Input: part model. Units: mm. Frame: model coordinates. A direction names the side the tool comes from. Coordinates: 2 decimals unless noted, no trailing zeros. Write each loop counter-clockwise with the first axis right and the second up, starting at its lowest first coordinate (ties: lowest second). Pieces come first, ordered by that corner, then holes. Notation, with made-up numbers: M -22,66.25 L -14,66.25 A12 cw -14,74.25 Z; hole C 79,27.25 d8. An arc over 180 degrees is marked long. Answer as a JSON object with one key per item and string values. Group by question number.
from build123d import *

# Parameters (mm, degrees)
F0_W      = 125
F0_H      = 200
F1_DEPTH  = 50
F2_W      = 50
F2_H      = 70
F3_DEPTH  = 35
F5_DEPTH  = 50
F6_R      = 20
F7_DEPTH  = 50.001
F9_DEPTH  = 30
F10_W     = 75
F10_H     = 25
F11_DEPTH = 200.001
F12_W     = 40
F12_H     = 50
F13_DEPTH = 20
F15_DEPTH = 40


with BuildPart() as f1:
    # F0 (on Top) → F1 (new body)
    with BuildSketch(Plane.XY):
        with Locations((-0.529949, 21.220052)):
            Rectangle(F0_W, F0_H)
    extrude(amount=F1_DEPTH)

    # F2 (on face) → F3 (join)
    with BuildSketch(Plane.XY.offset(50)):
        with Locations((-38.029949, 86.220052)):
            Rectangle(F2_W, F2_H)
    extrude(amount=F3_DEPTH)

    # F4 (on face) → F5 (join)
    with BuildSketch(Plane.YZ.offset(-13.029949)):
        with BuildLine():
            Line((51.220052, 85), (121.220052, 85))
            ThreePointArc((121.220052, 85), (86.220052, 120), (51.220052, 85))
        make_face()
    extrude(amount=-F5_DEPTH)

    # F6 (on face) → F7 (cut, through all)
    with BuildSketch(Plane.YZ.offset(-13.029949)):
        with Locations((86.220052, 85)):
            Circle(F6_R)
    extrude(amount=-F7_DEPTH, mode=Mode.SUBTRACT)

    # F8 (on face) → F9 (join)
    with BuildSketch(Plane(origin=(-63.029949, 0, 0), x_dir=(0, -1, 0), z_dir=(-1, 0, 0))):
        with BuildLine():
            Line((-51.220052, 50), (8.779948, 50))
            Line((8.779948, 50), (-63.512735, 111.634146))
            ThreePointArc((-63.512735, 111.634146), (-54.441474, 99.667036), (-51.220052, 85))
            Line((-51.220052, 85), (-51.220052, 50))
        make_face()
    extrude(amount=-F9_DEPTH)

    # F10 (on face) → F11 (cut, through all)
    with BuildSketch(Plane.XZ.offset(78.779948)):
        with Locations((-0.529949, 12.5)):
            Rectangle(F10_W, F10_H)
    extrude(amount=-F11_DEPTH, mode=Mode.SUBTRACT)

    # F12 (on face) → F13 (cut)
    with BuildSketch(Plane.YZ.offset(61.970051)):
        with Locations((21.220052, 25)):
            Rectangle(F12_W, F12_H)
    extrude(amount=-F13_DEPTH, mode=Mode.SUBTRACT)

    # F14 (on face) → F15 (join)
    with BuildSketch(Plane.XZ.offset(-41.220052)):
        Polygon((61.970051, 0), (41.970051, 50), (41.970051, 0), align=None)
    extrude(amount=F15_DEPTH)


solid = f1.part
Q1. Section D-D, the plane x = 20. Return the cut outline in (y, z).
Q2. Pin query (flat end, axial travel): pin 1 Ø1.5 at (y, z) = (49.5, 86.5) entering from +X; pin 2 Ø1 at (x, y) = (37, 65) entering from +Z; pin 3 Ø1.5 at (x, y) = (-18, 75.5) entering from +Z. Return the tip coordinate at first contact, or that it passes through.
Q3. Section C-C, the plane y = -65. Return the cut outline in (x, z).
Q4. Section A-A, the plane x = -46. Return the cut outline in (y, z).
Q5. Access query for faces 4 (the flat face through (52.11, 21.5, 24.65)), 5 (the flat face through (-13.03, 101, 70)), 6 (the flat face through (36.97, 20, 12)), 7 (the flat face through (-33.03, 30, 65)). Directions: +Z, -Z, +X, -X, +Y, -Y. A direction counts if a zero-diameter tool reaches every point of the face in a straight line with its end or side. Return the directions, or none.
Q6. Section B-B, the plane z = 81. Return the cut outline in (x, y), and give its area (3 significant figures).
Q7. Line query: line 1 (X direction, y = 62.5, z = 21); line 2 (Y direction, x = 49, z = 49.5); line 3 (Z direction, x = 14, y = 39). Output: solid intervals per line, ascending. Write a range as from..to.
Q8. Draft query along Z for faces 1 (the cylindrical face through (-37.68, 81.884, 65.476)), 2 (the flat face through (-1, 20, 25)), 3 (the flat face through (-48.24, 26.859, 80.384)). Return one class per face: released by +Z, released by -Z, zero draft, split by the parting line, or undercut.
Filled in:
{
 "1": {"outline": "M -78.78,25 L 121.22,25 L 121.22,50 L -78.78,50 Z"},
 "2": {"pin 1": "x = -33.03", "pin 2": "z = 50", "pin 3": "z = 118.55"},
 "3": {"outline": "M -63.03,0 L -38.03,0 L -38.03,25 L 36.97,25 L 36.97,0 L 61.97,0 L 61.97,50 L -63.03,50 Z"},
 "4": {"outline": "M -78.78,0 L 121.22,0 L 121.22,85 A35 ccw 63.51,111.63 L -8.78,50 L -78.78,50 Z; hole C 86.22,85 d40"},
 "5": {"face 4": "+Z, +X", "face 5": "+Z, +X, +Y, -Y", "face 6": "-Z, +Y, -Y", "face 7": "+Z, +X, -Y"},
 "6": {"outline": "M -63.03,27.58 L -33.03,27.58 L -33.03,51.22 L -13.03,51.22 L -13.03,66.62 L -63.03,66.62 Z; M -63.03,105.82 L -13.03,105.82 L -13.03,121.22 L -63.03,121.22 Z", "area": "2,250 mm^2"},
 "7": {"line 1": "-63.03..-38.03, 36.97..61.97", "line 2": "-78.78..1.22, 41.22..121.22", "line 3": "25..50"},
 "8": {"face 1": "undercut", "face 2": "released by -Z", "face 3": "released by +Z"}
}
